Build history of the part. All positions in model axes, mm. Give positions to 0.01 mm unless a question says otherwise; leave off trailing zeros. Write each loop counter-clockwise with the first axis right and the second up, starting at its lowest first coordinate (ties: lowest second). Pieces come first, ordered by that corner, then holes.
from build123d import *

# Parameters (mm, degrees)
SKETCH1_W           = 3.429
SKETCH1_H           = 6.858
SKETCH1_W_2         = 15.24
SKETCH1_H_2         = 4.191
BOSS_EXTRUDE1_DEPTH = 3.175


with BuildPart() as part:
    # Sketch1 → Boss-Extrude1 (new body)
    with BuildSketch(Plane(origin=(0, 0, 0), x_dir=(1, 0, 0), z_dir=(0, 1, 0))):
        with BuildLine():
            Line((-24.892, -15.875), (24.892, -15.875))
            ThreePointArc((24.892, -15.875), (29.083, -20.066), (33.274, -15.875))
            Line((33.274, -15.875), (33.274, 15.875))
            Line((33.274, 15.875), (-33.274, 15.875))
            Line((-33.274, 15.875), (-33.274, -15.875))
            ThreePointArc((-33.274, -15.875), (-29.083, -20.066), (-24.892, -15.875))
        make_face()
        with Locations((29.3497, 9.906)):
            Rectangle(SKETCH1_W, SKETCH1_H, mode=Mode.SUBTRACT)
        with Locations((29.3497, -9.906)):
            Rectangle(SKETCH1_W, SKETCH1_H, mode=Mode.SUBTRACT)
        with Locations((-29.3497, -9.906)):
            Rectangle(SKETCH1_W, SKETCH1_H, mode=Mode.SUBTRACT)
        with Locations((-29.3497, 9.906)):
            Rectangle(SKETCH1_W, SKETCH1_H, mode=Mode.SUBTRACT)
        with Locations((-0.3048, -9.3345)):
            Rectangle(SKETCH1_W_2, SKETCH1_H_2, mode=Mode.SUBTRACT)
    extrude(amount=BOSS_EXTRUDE1_DEPTH)


solid = part.part
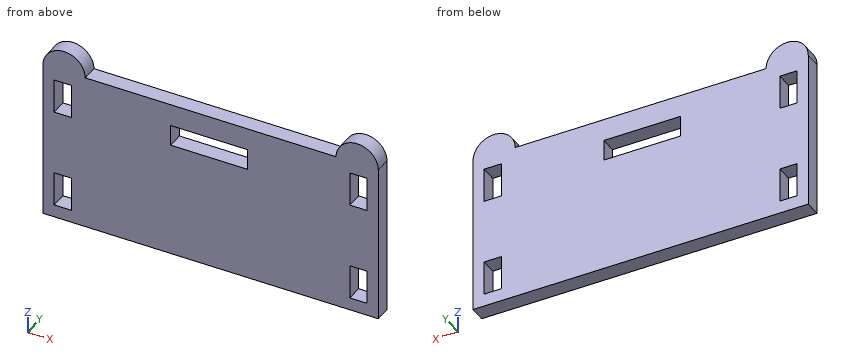
1. Saw through at A-A on y = 1.85. Give the cut face in (x, z) (3 decimals), plus the area to 3 significant figures.
2. Drop a flat-ended pin along its axis: pin 1 (1 mm diameter, centred on x = -7.5, y = 2, fed in from +Z) (3 decimals). Give the stop position or say it passes through.
3. Drill centre lines: line 1 along X through (y, z) = (0.25, -9); line 2 along X through (y, z) = (0.9, 7.5); line 3 along Z through (x, y) = (-6, 2.7) (3 decimals). Where is each one in solid material? Low to high.
4. Saw through at C-C on z = 9. Give the cut face in (x, y) (3 decimals), plus the area to 3 significant figures.
5. Saw through at B-B on x = -2. Give the cut face in (y, z) (3 decimals).
6. Saw through at D-D on x = 9.5. Give the cut face in (y, z) (3 decimals).
Outcome:
1. outline: (-33.274, -15.875) - (33.274, -15.875) - (33.274, 15.875) arc R4.191 ccw to (24.892, 15.875) - (-24.892, 15.875) arc R4.191 ccw to (-33.274, 15.875) - close; hole (-31.064, -13.335) - (-27.635, -13.335) - (-27.635, -6.477) - (-31.064, -6.477) - close; hole (-31.064, 6.477) - (-27.635, 6.477) - (-27.635, 13.335) - (-31.064, 13.335) - close; hole (-7.925, 7.239) - (7.315, 7.239) - (7.315, 11.43) - (-7.925, 11.43) - close; hole (27.635, -13.335) - (31.064, -13.335) - (31.064, -6.477) - (27.635, -6.477) - close; hole (27.635, 6.477) - (31.064, 6.477) - (31.064, 13.335) - (27.635, 13.335) - close
1. area: 2,010 mm2
2. pin 1: stops at z = 15.875
3. line 1: x = -33.27 to -31.06, -27.64 to 27.64, 31.06 to 33.27
3. line 2: x = -33.27 to -31.06, -27.64 to -7.92, 7.32 to 27.64, 31.06 to 33.27
3. line 3: z = -15.875 to 7.239, 11.43 to 15.875
4. outline: (-33.274, 0) - (-31.064, 0) - (-31.064, 3.175) - (-33.274, 3.175) - close; (-27.635, 0) - (-7.925, 0) - (-7.925, 3.175) - (-27.635, 3.175) - close; (7.315, 0) - (27.635, 0) - (27.635, 3.175) - (7.315, 3.175) - close; (31.064, 0) - (33.274, 0) - (33.274, 3.175) - (31.064, 3.175) - close
4. area: 141 mm2
5. outline: (0, -15.875) - (3.175, -15.875) - (3.175, 7.239) - (0, 7.239) - close; (0, 11.43) - (3.175, 11.43) - (3.175, 15.875) - (0, 15.875) - close
6. outline: (0, -15.875) - (3.175, -15.875) - (3.175, 15.875) - (0, 15.875) - close
